Design review of the part built by this model. Coordinates are the model's own, in mm. Face numbers are marked on the shaded views. Give positions to 0.01 mm unless a question says otherwise; leave off trailing zeros. Order: outer loops, then holes, each group sorted by start corner. A loop starts at its lowest first (then second) coordinate and runs counter-clockwise, first axis right, second up. Notation, with made-up numbers: (-15.75, 12) -> (5.25, 12) arc R8 ccw to (5.25, 20) -> close; hole circle Ø10 at (82.25, 86.5). An arc over 180 degrees is marked (long way). One line per item, written item: value. Start each with the question number.
1) Consider section A-A (x = 15). State the section outline as (y, z) points, plus the area to 3 significant figures.
2) For pin 1 (1.8 mm diameter, centred on x = 15, z = -3, fed in from -Y), flat-tipped, find the tip position at first contact; note if it passes through.
3) Consider section B-B (y = 1). State how many separate pieces and enclosed holes the cut face has, plus the area to 3 significant figures.
4) Consider section C-C (z = 10). State the section outline as (x, y) points, plus the area to 3 significant figures.
5) Consider section D-D (z = 1). State the section outline as (x, y) points, plus the area to 3 significant figures.
6) The part is to be moulded in two halves that separate along X. For the marked faces 1, 2 and 3, say which applies: released by +X, released by -X, zero draft, split by the parting line, or undercut.
7) Wall thickness on line 1 along X through (y, z) = (0.75, -3); line 2 along Z through (x, y) = (12.75, 1.4): over which ranges is each line inside the solid? List them lowest first. Write a range as from..to.
from build123d import *

# Parameters (mm, degrees)
BOSS_EXTRUDE1_DEPTH = 2
SKETCH2_R           = 1.1
CUT_EXTRUDE1_DEPTH  = 2
FILLET1_R           = 3


with BuildPart() as part:
    # Sketch1 → Boss-Extrude1 (new body)
    with BuildSketch(Plane(origin=(0, 0, 0), x_dir=(1, 0, 0), z_dir=(0, 1, 0))):
        Polygon((-6, 6), (-6, -14), (0, -14), (0, 0), (19, 0), (19, 6), align=None)
    extrude(amount=BOSS_EXTRUDE1_DEPTH)

    # Sketch2 → Cut-Extrude1 (cut)
    with BuildSketch(Plane(origin=(0, 2, 0), x_dir=(1, 0, 0), z_dir=(0, 1, 0))):
        with Locations(Location((-3, -10, 0), (0, 0, 270))):
            Circle(SKETCH2_R)
        with Locations(Location((15, 3, 0), (0, 0, 270))):
            Circle(SKETCH2_R)
    extrude(amount=-CUT_EXTRUDE1_DEPTH, mode=Mode.SUBTRACT)

    # Fillet1
    fillet1_edges = [part.edges().sort_by_distance(p)[0] for p in [
        (19, 1, -6),
        (19, 1, 0),
        (-6, 1, 14),
        (0, 1, 14),
    ]]
    fillet(fillet1_edges, radius=FILLET1_R - 0.0001)  # a hair under: the kernel refuses the full size


solid = part.part
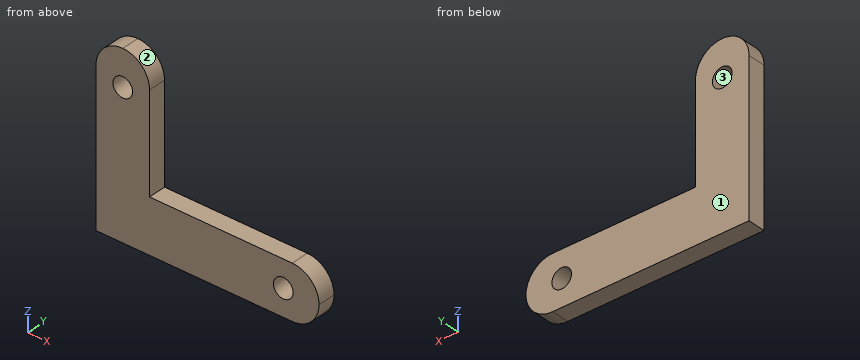
Checked values:
1. outline: (0, -6) -> (2, -6) -> (2, -4.1) -> (0, -4.1) -> close; (0, -1.9) -> (2, -1.9) -> (2, 0) -> (0, 0) -> close
1. area: 7.60 mm^2
2. pin 1: passes through
3. separate pieces: 1
3. enclosed holes: 2
3. area: 219 mm^2
4. outline: (-6, 0) -> (-4.1, 0) -> (-4.1, 2) -> (-6, 2) -> close; (-1.9, 0) -> (0, 0) -> (0, 2) -> (-1.9, 2) -> close
4. area: 7.60 mm^2
5. outline: (-6, 0) -> (0, 0) -> (0, 2) -> (-6, 2) -> close
5. area: 12.0 mm^2
6. face 1: zero draft
6. face 2: released by +X
6. face 3: undercut
7. line 1: x = -6..13.9, 16.1..19
7. line 2: z = -6..0
